```python
from build123d import *

# Parameters (mm, degrees)
F0_R     = 13.55
F1_DEPTH = 1.25
F0_R_2   = 12.55
F2_DEPTH = 4.9
F0_R_3   = 1.5
F0_R_4   = 8.5
F3_DEPTH = 1
F0_R_5   = 7.7
F4_DEPTH = 4.9
F5_R     = 7.7
F5_R_2   = 6.2
F6_DEPTH = 2.4


with BuildPart() as f1:
    # F0 (on Front) → F1 (new body, symmetric)
    with BuildSketch(Plane.XZ):
        with BuildLine():
            Line((4.1411047216, 15.4548132206), (2.0884190755, 15.863117782))
            Line((2.0884190755, 15.863117782), (1.0442095378, 15.931558891))
            Line((1.0442095378, 15.931558891), (1.021095107, 15.9673844064))
            ThreePointArc((1.021095107, 15.9673844064), (0, 16), (-1.021095107, 15.9673844064))
            Line((-1.021095107, 15.9673844064), (-1.0442095378, 15.931558891))
            Line((-1.0442095378, 15.931558891), (-2.0884190755, 15.863117782))
            Line((-2.0884190755, 15.863117782), (-4.1411047216, 15.4548132206))
            Line((-4.1411047216, 15.4548132206), (-5.1320198197, 15.1184428704))
            Line((-5.1320198197, 15.1184428704), (-5.1670846004, 15.1426958212))
            ThreePointArc((-5.1670846004, 15.1426958212), (-6.1229349178, 14.7820725202), (-7.0538223407, 14.3611834605))
            Line((-7.0538223407, 14.3611834605), (-7.0614674589, 14.3192394904))
            Line((-7.0614674589, 14.3192394904), (-8, 13.8564064606))
            Line((-8, 13.8564064606), (-9.7401828641, 12.6936534447))
            Line((-9.7401828641, 12.6936534447), (-10.5269456816, 12.0036809718))
            Line((-10.5269456816, 12.0036809718), (-10.5686225172, 12.012669066))
            ThreePointArc((-10.5686225172, 12.012669066), (-11.313708499, 11.313708499), (-12.012669066, 10.5686225172))
            Line((-12.012669066, 10.5686225172), (-12.0036809718, 10.5269456816))
            Line((-12.0036809718, 10.5269456816), (-12.6936534447, 9.7401828641))
            Line((-12.6936534447, 9.7401828641), (-13.8564064606, 8))
            Line((-13.8564064606, 8), (-14.3192394904, 7.0614674589))
            Line((-14.3192394904, 7.0614674589), (-14.3611834605, 7.0538223407))
            ThreePointArc((-14.3611834605, 7.0538223407), (-14.7820725202, 6.1229349178), (-15.1426958212, 5.1670846004))
            Line((-15.1426958212, 5.1670846004), (-15.1184428704, 5.1320198197))
            Line((-15.1184428704, 5.1320198197), (-15.4548132206, 4.1411047216))
            Line((-15.4548132206, 4.1411047216), (-15.863117782, 2.0884190755))
            Line((-15.863117782, 2.0884190755), (-15.931558891, 1.0442095378))
            Line((-15.931558891, 1.0442095378), (-15.9673844064, 1.021095107))
            ThreePointArc((-15.9673844064, 1.021095107), (-16, 0), (-15.9673844064, -1.021095107))
            Line((-15.9673844064, -1.021095107), (-15.931558891, -1.0442095378))
            Line((-15.931558891, -1.0442095378), (-15.863117782, -2.0884190755))
            Line((-15.863117782, -2.0884190755), (-15.4548132206, -4.1411047216))
            Line((-15.4548132206, -4.1411047216), (-15.1184428704, -5.1320198197))
            Line((-15.1184428704, -5.1320198197), (-15.1426958212, -5.1670846004))
            ThreePointArc((-15.1426958212, -5.1670846004), (-14.7820725202, -6.1229349178), (-14.3611834605, -7.0538223407))
            Line((-14.3611834605, -7.0538223407), (-14.3192394904, -7.0614674589))
            Line((-14.3192394904, -7.0614674589), (-13.8564064606, -8))
            Line((-13.8564064606, -8), (-12.6936534447, -9.7401828641))
            Line((-12.6936534447, -9.7401828641), (-12.0036809718, -10.5269456816))
            Line((-12.0036809718, -10.5269456816), (-12.012669066, -10.5686225172))
            ThreePointArc((-12.012669066, -10.5686225172), (-11.313708499, -11.313708499), (-10.5686225172, -12.012669066))
            Line((-10.5686225172, -12.012669066), (-10.5269456816, -12.0036809718))
            Line((-10.5269456816, -12.0036809718), (-9.7401828641, -12.6936534447))
            Line((-9.7401828641, -12.6936534447), (-8, -13.8564064606))
            Line((-8, -13.8564064606), (-7.0614674589, -14.3192394904))
            Line((-7.0614674589, -14.3192394904), (-7.0538223407, -14.3611834605))
            ThreePointArc((-7.0538223407, -14.3611834605), (-6.1229349178, -14.7820725202), (-5.1670846004, -15.1426958212))
            Line((-5.1670846004, -15.1426958212), (-5.1320198197, -15.1184428704))
            Line((-5.1320198197, -15.1184428704), (-4.1411047216, -15.4548132206))
            Line((-4.1411047216, -15.4548132206), (-2.0884190755, -15.863117782))
            Line((-2.0884190755, -15.863117782), (-1.0442095378, -15.931558891))
            Line((-1.0442095378, -15.931558891), (-1.021095107, -15.9673844064))
            ThreePointArc((-1.021095107, -15.9673844064), (0, -16), (1.021095107, -15.9673844064))
            Line((1.021095107, -15.9673844064), (1.0442095378, -15.931558891))
            Line((1.0442095378, -15.931558891), (2.0884190755, -15.863117782))
            Line((2.0884190755, -15.863117782), (4.1411047216, -15.4548132206))
            Line((4.1411047216, -15.4548132206), (5.1320198197, -15.1184428704))
            Line((5.1320198197, -15.1184428704), (5.1670846004, -15.1426958212))
            ThreePointArc((5.1670846004, -15.1426958212), (6.1229349178, -14.7820725202), (7.0538223407, -14.3611834605))
            Line((7.0538223407, -14.3611834605), (7.0614674589, -14.3192394904))
            Line((7.0614674589, -14.3192394904), (8, -13.8564064606))
            Line((8, -13.8564064606), (9.7401828641, -12.6936534447))
            Line((9.7401828641, -12.6936534447), (10.5269456816, -12.0036809718))
            Line((10.5269456816, -12.0036809718), (10.5686225172, -12.012669066))
            ThreePointArc((10.5686225172, -12.012669066), (11.313708499, -11.313708499), (12.012669066, -10.5686225172))
            Line((12.012669066, -10.5686225172), (12.0036809718, -10.5269456816))
            Line((12.0036809718, -10.5269456816), (12.6936534447, -9.7401828641))
            Line((12.6936534447, -9.7401828641), (13.8564064606, -8))
            Line((13.8564064606, -8), (14.3192394904, -7.0614674589))
            Line((14.3192394904, -7.0614674589), (14.3611834605, -7.0538223407))
            ThreePointArc((14.3611834605, -7.0538223407), (14.7820725202, -6.1229349178), (15.1426958212, -5.1670846004))
            Line((15.1426958212, -5.1670846004), (15.1184428704, -5.1320198197))
            Line((15.1184428704, -5.1320198197), (15.4548132206, -4.1411047216))
            Line((15.4548132206, -4.1411047216), (15.863117782, -2.0884190755))
            Line((15.863117782, -2.0884190755), (15.931558891, -1.0442095378))
            Line((15.931558891, -1.0442095378), (15.9673844064, -1.021095107))
            ThreePointArc((15.9673844064, -1.021095107), (15.9918440229, -0.5108079371), (16, 0))
            ThreePointArc((16, 0), (15.9918440229, 0.5108079371), (15.9673844064, 1.021095107))
            Line((15.9673844064, 1.021095107), (15.931558891, 1.0442095378))
            Line((15.931558891, 1.0442095378), (15.863117782, 2.0884190755))
            Line((15.863117782, 2.0884190755), (15.4548132206, 4.1411047216))
            Line((15.4548132206, 4.1411047216), (15.1184428704, 5.1320198197))
            Line((15.1184428704, 5.1320198197), (15.1426958212, 5.1670846004))
            ThreePointArc((15.1426958212, 5.1670846004), (14.7820725202, 6.1229349178), (14.3611834605, 7.0538223407))
            Line((14.3611834605, 7.0538223407), (14.3192394904, 7.0614674589))
            Line((14.3192394904, 7.0614674589), (13.8564064606, 8))
            Line((13.8564064606, 8), (12.6936534447, 9.7401828641))
            Line((12.6936534447, 9.7401828641), (12.0036809718, 10.5269456816))
            Line((12.0036809718, 10.5269456816), (12.012669066, 10.5686225172))
            ThreePointArc((12.012669066, 10.5686225172), (11.313708499, 11.313708499), (10.5686225172, 12.012669066))
            Line((10.5686225172, 12.012669066), (10.5269456816, 12.0036809718))
            Line((10.5269456816, 12.0036809718), (9.7401828641, 12.6936534447))
            Line((9.7401828641, 12.6936534447), (8, 13.8564064606))
            Line((8, 13.8564064606), (7.0614674589, 14.3192394904))
            Line((7.0614674589, 14.3192394904), (7.0538223407, 14.3611834605))
            ThreePointArc((7.0538223407, 14.3611834605), (6.1229349178, 14.7820725202), (5.1670846004, 15.1426958212))
            Line((5.1670846004, 15.1426958212), (5.1320198197, 15.1184428704))
            Line((5.1320198197, 15.1184428704), (4.1411047216, 15.4548132206))
        make_face()
        Circle(F0_R, mode=Mode.SUBTRACT)
    extrude(amount=F1_DEPTH, both=True)

    # F0 (on Front) → F2 (join, symmetric)
    with BuildSketch(Plane.XZ):
        Circle(F0_R)
        Circle(F0_R_2, mode=Mode.SUBTRACT)
    extrude(amount=F2_DEPTH, both=True)

    # F0 (on Front) → F3 (join, symmetric)
    with BuildSketch(Plane.XZ):
        Circle(F0_R_2)
        with Locations((-2.056837265, -10.3404192113)):
            Circle(F0_R_3, mode=Mode.SUBTRACT)
        with Locations((-10.3404192113, -2.056837265)):
            Circle(F0_R_3, mode=Mode.SUBTRACT)
        with Locations((-5.8573769667, -8.7661841225)):
            Circle(F0_R_3, mode=Mode.SUBTRACT)
        with Locations((-8.7661841225, -5.8573769667)):
            Circle(F0_R_3, mode=Mode.SUBTRACT)
        with Locations((2.056837265, -10.3404192113)):
            Circle(F0_R_3, mode=Mode.SUBTRACT)
        with Locations((5.8573769667, -8.7661841225)):
            Circle(F0_R_3, mode=Mode.SUBTRACT)
        with Locations((8.7661841225, -5.8573769667)):
            Circle(F0_R_3, mode=Mode.SUBTRACT)
        with Locations((10.3404192113, -2.056837265)):
            Circle(F0_R_3, mode=Mode.SUBTRACT)
        with Locations((-10.3404192113, 2.056837265)):
            Circle(F0_R_3, mode=Mode.SUBTRACT)
        with Locations((-8.7661841225, 5.8573769667)):
            Circle(F0_R_3, mode=Mode.SUBTRACT)
        with Locations((-5.8573769667, 8.7661841225)):
            Circle(F0_R_3, mode=Mode.SUBTRACT)
        with Locations((-2.056837265, 10.3404192113)):
            Circle(F0_R_3, mode=Mode.SUBTRACT)
        Circle(F0_R_4, mode=Mode.SUBTRACT)
        with Locations((8.7661841225, 5.8573769667)):
            Circle(F0_R_3, mode=Mode.SUBTRACT)
        with Locations((5.8573769667, 8.7661841225)):
            Circle(F0_R_3, mode=Mode.SUBTRACT)
        with Locations((10.3404192113, 2.056837265)):
            Circle(F0_R_3, mode=Mode.SUBTRACT)
        with Locations((2.056837265, 10.3404192113)):
            Circle(F0_R_3, mode=Mode.SUBTRACT)
    extrude(amount=F3_DEPTH, both=True)

    # F0 (on Front) → F4 (join, symmetric)
    with BuildSketch(Plane.XZ):
        Circle(F0_R_4)
        Circle(F0_R_5, mode=Mode.SUBTRACT)
    extrude(amount=F4_DEPTH, both=True)

    # F5 (on face) → F6 (join)
    with BuildSketch(Plane(origin=(0, 4.9, 0), x_dir=(-1, 0, 0), z_dir=(0, 1, 0))):
        Circle(F5_R)
        Circle(F5_R_2, mode=Mode.SUBTRACT)
    extrude(amount=-F6_DEPTH)


solid = f1.part
```
Part model, mm, in its own coordinate system. A direction names the side the tool comes from. Give positions to 0.01 mm unless a question says otherwise; leave off trailing zeros. Write each loop counter-clockwise with the first axis right and the second up, starting at its lowest first coordinate (ties: lowest second). Pieces come first, ordered by that corner, then holes. Notation, with made-up numbers: M 84,9 L 106,9 A13 cw 106,33 Z; hole C -26,-34.75 d7. An arc over 180 degrees is marked long. Use CSV: the item, a comma, the result in double quotes.
Item 1: Slice it at A-A on y = -1.75. Write the cut outline in (x, z), plus the area to 3 significant figures.
Taken from the geometry:
outline,"C 0,0 d27.1; C 0,0 d17; hole C 0,0 d25.1; hole C 0,0 d15.4"
area,"123 mm²"
Item 2: Pull direction X, two halves, no side cores. Call faces 4 (the face through (-1, -4.9, 8)), 5 (the face through (13.28, -0.02, 8.86)), 6 (the face through (11.59, 2.98, -4.81)), 7 (the face through (-6.11, -0.018, 14.788)): +X half, -X half, draft (parallel to the pull), parting line (faces both ways), or undercut.
Taken from the geometry:
face 4,"draft"
face 5,"+X half"
face 6,"undercut"
face 7,"-X half"
Item 3: Slice it at B-B on x = -11. Write the cut outline in (y, z).
Taken from the geometry:
outline,"M -4.9,-7.91 L -1.25,-7.91 L -1.25,-11.62 L 1.25,-11.62 L 1.25,-7.91 L 4.9,-7.91 L 4.9,-6.04 L 1,-6.04 L 1,-3.4 L -1,-3.4 L -1,-6.04 L -4.9,-6.04 Z; M -4.9,6.04 L -1,6.04 L -1,3.4 L 1,3.4 L 1,6.04 L 4.9,6.04 L 4.9,7.91 L 1.25,7.91 L 1.25,11.62 L -1.25,11.62 L -1.25,7.91 L -4.9,7.91 Z; M -1,-0.71 L 1,-0.71 L 1,0.71 L -1,0.71 Z"
Item 4: Which spindle directions (+Z, -Z, +X, -X, +Y, -Y) get a long thin tool onto all of the face, cutting with end or side? Do faces 1 (the face through (-5.05, 0.01, 10.03)), 2 (the face through (-12, 1.25, 7)), 3 (the face through (11.59, -2.92, -4.81)). Say none if no direction does.
Taken from the geometry:
face 1,"+Y, -Y"
face 2,"+Y"
face 3,"-Y"
Item 5: Drill centre lines: probe 1 along Z at (x, y) = (-2, 0.5); probe 2 along X at (y, z) = (-3.5, -1); probe 3 along X at (y, z) = (0.5, 11.5). Where is each one in solid material? Low to high.
Taken from the geometry:
probe 1,"z = -15.87 to -11.84, -8.84 to -7.44, 7.44 to 8.84, 11.84 to 15.87"
probe 2,"x = -13.51 to -12.51, -8.44 to -7.63, 7.63 to 8.44, 12.51 to 13.51"
probe 3,"x = -11.12 to -3.01, -1.11 to 1.11, 3.01 to 11.12"
Item 6: Slice it at C-C on z = 2.5. State how many separate pieces and enclosed holes the cut face has, plus the area to 3 significant figures.
Taken from the geometry:
separate pieces,"4"
enclosed holes,"0"
area,"61.7 mm²"
Item 7: Pin check, flat tips, straight feed: P1, Ø3, axis at x = -3, y = 0, coming from the -Z side; P2, Ø7.5, axis at x = -2.5, z = 5, coming from the -Y side; P3, Ø3.5, axis at x = -5.86, z = 8.77, coming from the +Y side; P4, Ø3.5, axis at x = -10.34, z = 2.06, coming from the -Y side. Stop position of each tip, or through.
Taken from the geometry:
P1,"stops at z = -15.9"
P2,"stops at y = -4.9"
P3,"stops at y = 1"
P4,"stops at y = -1"
